Input: dimensioned drawing with shaded views. Units: mm. Origin: part minimum x, y, z. Coordinates: 2 decimals unless noted, no trailing zeros. Loops run counter-clockwise (first coordinate to the right, second up) from the corner with the lowest first, then second, coordinate; pieces in that order, holes last.
(1) Section A-A, the plane x = 30. Return loops of the section in (y, z) (1 decimal).
(2) Contact query for flat-ended pins moving along their axis: P1, Ø3, axis at x = 21, y = 52.5, coming from the -Z side; P2, Ø2.5, axis at x = 30, y = 14.17, coming from the -Z side. Output: stop coordinate, or through.
(3) Line query: L1, parallel to Y at x = 30, z = 0.5 (1 decimal); L2, parallel to Y at x = 31.5, z = 1.65 (1 decimal). Output: solid intervals per line, ascending.
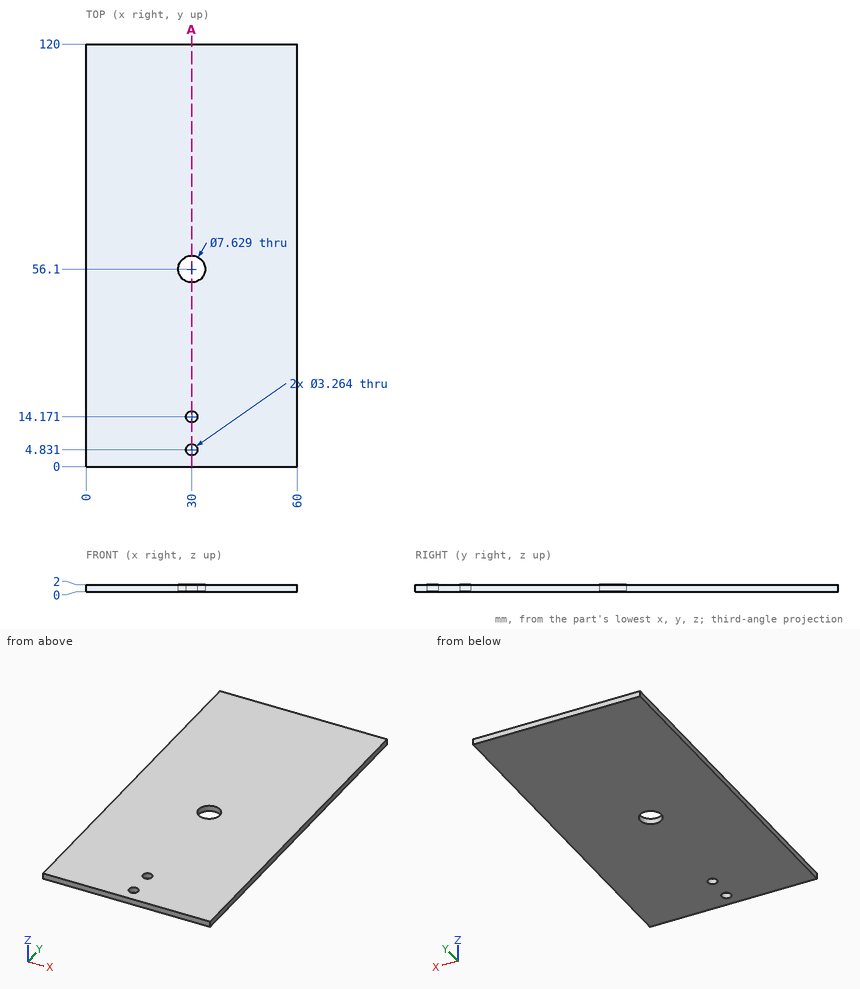
Report:
1. outline: (0, 0) - (3.2, 0) - (3.2, 2) - (0, 2) - close; (6.5, 0) - (12.5, 0) - (12.5, 2) - (6.5, 2) - close; (15.8, 0) - (52.3, 0) - (52.3, 2) - (15.8, 2) - close; (59.9, 0) - (120, 0) - (120, 2) - (59.9, 2) - close
2. P1: stops at z = 0
2. P2: passes through
3. L1: y = 0 to 3.2, 6.5 to 12.5, 15.8 to 52.3, 59.9 to 120
3. L2: y = 0 to 4.2, 5.5 to 13.5, 14.8 to 52.6, 59.6 to 120
